Geometry: see drawing. Coordinates: mm, zero at the bounding-box minimum. Round coordinates to 2 decimals unless told otherwise and drop trailing zeros. Loops run counter-clockwise (first coordinate to the right, second up) from the corner with the lowest first, then second, coordinate; pieces in that order, holes last.
(1) Cut plane B-B, the plane y = 2.3. Give the number of separate pieces and of enclosed holes in the cut face, and give its area (3 significant figures).
(2) Cut plane A-A, the plane x = 172.5. Output: boundary loops of the cut face in (y, z).
(3) First-contact query: pin 1 Ø3 at (x, z) = (61.75, 100) entering from +Y. Flat tip, straight axial feed; report the tip coordinate or a pass-through.
(4) Line query: line 1 (Z direction, x = 71.5, y = 3.2); line 2 (Z direction, x = 61.75, y = 2.6); line 3 (X direction, y = 1.35, z = 189.5). Output: solid intervals per line, ascending.
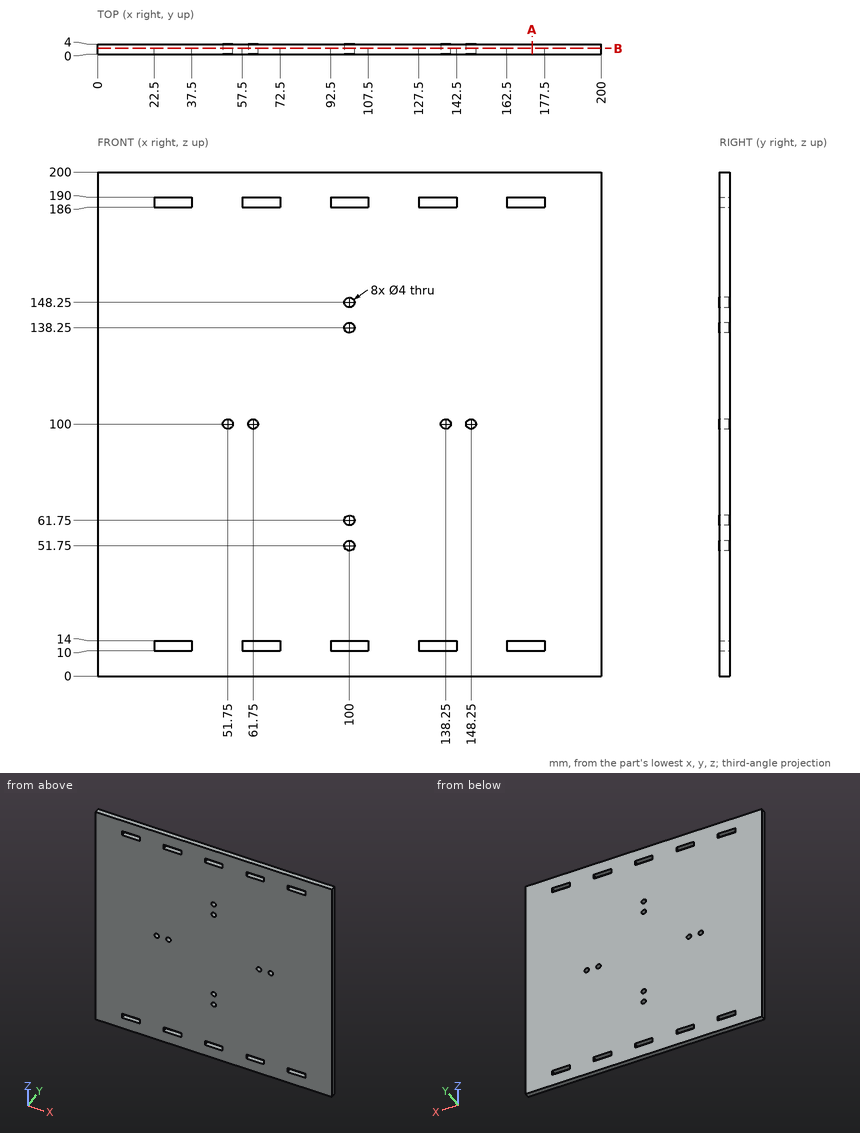
Reported:
1. separate pieces: 1
1. enclosed holes: 18
1. area: 39,300 mm2
2. outline: (0, 0) - (4, 0) - (4, 10) - (0, 10) - close; (0, 14) - (4, 14) - (4, 186) - (0, 186) - close; (0, 190) - (4, 190) - (4, 200) - (0, 200) - close
3. pin 1: passes through
4. line 1: z = 0 to 10, 14 to 186, 190 to 200
4. line 2: z = 0 to 10, 14 to 98, 102 to 186, 190 to 200
4. line 3: x = 0 to 22.5, 37.5 to 57.5, 72.5 to 92.5, 107.5 to 127.5, 142.5 to 162.5, 177.5 to 200
